from build123d import *

# Parameters (mm, degrees)
ESQUISSE3_R                  = 35
ESQUISSE3_R_2                = 30
BOSS_EXTRU_3_DEPTH           = 250
ESQUISSE4_W                  = 124.19
ESQUISSE4_H                  = 26
ENL_V_MAT_EXTRU_1_DEPTH      = 100
ENL_V_MAT_EXTRU_2_DEPTH      = 100
ENL_V_MAT_EXTRU_2_DEPTH_BACK = 100
ESQUISSE6_R                  = 3


with BuildPart() as part:
    # Esquisse3 → Boss.-Extru.3 (new body)
    with BuildSketch(Plane(origin=(0, 0, 0), x_dir=(1, 0, 0), z_dir=(0, 1, 0))):
        with Locations(Location((0, 0, 0), (0, 0, 270))):
            Circle(ESQUISSE3_R)
        with Locations(Location((0, 0, 0), (0, 0, 270))):
            Circle(ESQUISSE3_R_2, mode=Mode.SUBTRACT)
    extrude(amount=BOSS_EXTRU_3_DEPTH)

    # Esquisse4 → Enlèv. mat.-Extru.1 (cut)
    with BuildSketch(Plane(origin=(0, 250, 0), x_dir=(1, 0, 0), z_dir=(0, 1, 0))):
        Rectangle(ESQUISSE4_W, ESQUISSE4_H)
    extrude(amount=-ENL_V_MAT_EXTRU_1_DEPTH, mode=Mode.SUBTRACT)

    # Esquisse6 → Enlèv. mat.-Extru.2 (cut, two sides: drawn at the far end of the back side and taken through both)
    with BuildSketch(Plane.XY.offset(-ENL_V_MAT_EXTRU_2_DEPTH_BACK)):
        with Locations(Location((0, 200, 0), (0, 0, 180))):
            Circle(ESQUISSE6_R)
    extrude(amount=ENL_V_MAT_EXTRU_2_DEPTH + ENL_V_MAT_EXTRU_2_DEPTH_BACK, mode=Mode.SUBTRACT)


solid = part.part
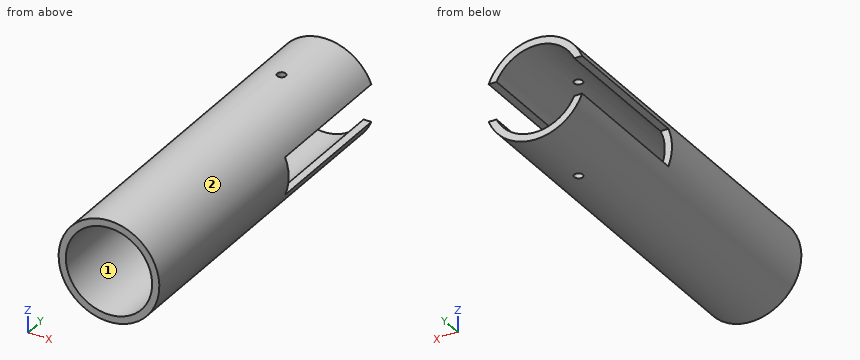
Model file for the job. Use its own axes, mm. Face numbers are marked on the shaded views. Round coordinates to 2 decimals unless told otherwise and drop trailing zeros. Loops run counter-clockwise (first coordinate to the right, second up) from the corner with the lowest first, then second, coordinate; pieces in that order, holes last. Notation, with made-up numbers: (41, 0) - (80, 0) arc R13 ccw to (80, 18) - close; hole circle Ø2 at (44, 31.25). An arc over 180 degrees is marked (long way). Write each question's results on one line, items separated by ' | '.
(1) Saw through at C-C, the plane y = 211.5. List the corners of the cut face in (x, z).
Answer below:
outline: (-32.5, -13) arc R35 ccw to (32.5, -13) - (27.04, -13) arc R30 cw to (-27.04, -13) - close; (-32.5, 13) - (-27.04, 13) arc R30 cw to (27.04, 13) - (32.5, 13) arc R35 ccw to start
(2) Mould opens along Z. For the marked faces 1 and 2 say: released by +Z, released by -Z, zero draft, split by the parting line, or undercut.
Answer below:
face 1: undercut | face 2: split by the parting line
(3) Wall check: L1, parallel to X at y = 24, z = 1.5; L2, parallel to Y at x = 0, z = 32; L3, parallel to Z at x = 13, y = 71. Give the ranges that are in metal, low to high.
Answer below:
L1: x = -34.97 to -29.96, 29.96 to 34.97 | L2: y = 0 to 197, 203 to 250 | L3: z = -32.5 to -27.04, 27.04 to 32.5
(4) Saw through at A-A, the plane x = 0. List the corners of the cut face in (y, z).
Answer below:
outline: (0, -35) - (197, -35) - (197, -30) - (0, -30) - close; (0, 30) - (197, 30) - (197, 35) - (0, 35) - close; (203, -35) - (250, -35) - (250, -30) - (203, -30) - close; (203, 30) - (250, 30) - (250, 35) - (203, 35) - close
(5) Saw through at D-D, the plane y = 45. List the corners of the cut face in (x, z).
Answer below:
outline: circle Ø70 at (0, 0); hole circle Ø60 at (0, 0)
(6) Saw through at B-B, the plane z = 0. List the corners of the cut face in (x, y), then the cut area to 3 significant figures.
Answer below:
outline: (-35, 0) - (-30, 0) - (-30, 150) - (-35, 150) - close; (30, 0) - (35, 0) - (35, 150) - (30, 150) - close | area: 1,500 mm^2
(7) Pin check, flat tips, straight feed: pin 1 (4 mm diameter, centred on x = -30, z = -6.5, fed in from +Y); pin 2 (6 mm diameter, centred on x = -4.5, y = 114, fed in from +Z); pin 3 (6 mm diameter, centred on x = -7.5, y = 120.5, fed in from -Z). Stop position of each tip, or through.
Answer below:
pin 1: stops at y = 150 | pin 2: stops at z = 34.97 | pin 3: stops at z = -34.71
